Source: CAD feature listing. Evaluate the final solid. Frame: model axes, mm. A direction names the side the tool comes from. Coordinates: 2 decimals unless noted, no trailing zeros. Write each loop counter-clockwise with the first axis right and the second up, starting at its lowest first coordinate (ties: lowest second). Pieces come first, ordered by that corner, then holes. Notation, with made-up numbers: (5.25, -20) -> (29.25, -20) arc R12 cw to (29.25, -4) -> close; hole circle Ø10 at (-22.75, 49). An arc over 180 degrees is marked (long way). Write item = value, one per line.
from build123d import *

# Parameters (mm, degrees)
CUT_EXTRUDE_START   = -0.5
CUT_EXTRUDE_1_DEPTH = 6.83442973
CHAMFER_1_SIZE      = 0.2


with BuildPart() as part:
    # 草图1 → 旋转1 (revolve)
    with BuildSketch(Plane.XY, mode=Mode.PRIVATE) as revolve_1_sk:
        with BuildLine():
            Line((1.2, 2.75), (1.9, 2.75))
            Line((1.9, 2.75), (1.9, 1.5))
            Line((1.9, 1.5), (6.9, 1.5))
            Line((6.9, 1.5), (6.9, 0))
            Line((6.9, 0), (0, 0))
            ThreePointArc((0, 0), (0.313064269, 1.500208319), (1.2, 2.75))
        make_face()
    revolve(revolve_1_sk.sketch.rotate(Axis((0, 0, 0), (1, 0, 0)), 90), axis=Axis((0, 0, 0), (1, 0, 0)))

    # 草图2 → 切除-拉伸1 (cut, through all)
    with BuildSketch(Plane(origin=(1.9, 0, 0), x_dir=(0, 0, -1), z_dir=(1, 0, 0)).offset(CUT_EXTRUDE_START)):
        Polygon((0.35, -0.35), (0.35, -1.5), (-0.35, -1.5), (-0.35, -0.35), (-1.5, -0.35), (-1.5, 0.35), (-0.35, 0.35), (-0.35, 1.5), (0.35, 1.5), (0.35, 0.35), (1.5, 0.35), (1.5, -0.35), align=None)
    extrude(amount=-CUT_EXTRUDE_1_DEPTH, mode=Mode.SUBTRACT)

    # 草图3 → 旋转3 (revolve)
    with BuildSketch(Plane.XY, mode=Mode.PRIVATE) as revolve_3_sk:
        Polygon((1.9, 0), (1.9, 2), (0.9, 2), (1.4, 0), align=None)
    revolve(revolve_3_sk.sketch.rotate(Axis((0, 0, 0), (1, 0, 0)), 13.134022306), axis=Axis((0, 0, 0), (1, 0, 0)))

    # 倒角1
    chamfer_1_edges = [part.edges().sort_by_distance(p)[0] for p in [
        (6.9, 0, -1.5),
    ]]
    chamfer(chamfer_1_edges, length=CHAMFER_1_SIZE)


solid = part.part
1) Cut plane B-B, the plane z = -1.95. Output: boundary loops of the cut face in (x, y).
Answer block:
outline = (1.2, -1.94) -> (1.9, -1.94) -> (1.9, 1.94) -> (1.2, 1.94) arc R3.2 ccw to start
2) Reachability of faces 4 (the cylindrical face through (4.33, -0.45, 1.43)), 5 (the flat face through (0.7, 0.9, -0.35)) from +Z, -Z, +X, -X, +Y, -Y: full face, straight path, thin tool, end or side. Return the list, or none.
Answer block:
face_4 = +X
face_5 = -X
3) Material intervals for probe 1 along Z at (x, y) = (3.25, 0.8); probe 2 along Z at (x, y) = (6.25, -1.05); probe 3 along X at (y, z) = (-0.3, 0.1), sorted ascending. Write a range as [from, to].
Answer block:
probe_1 = [-1.27, 1.27]
probe_2 = [-1.07, 1.07]
probe_3 = [1.32, 6.9]
4) Cut plane A-A, the plane x = 4. Output: boundary loops of the cut face in (y, z).
Answer block:
outline = circle Ø3 at (0, 0)
5) Pull-direction query (Y, two-part tool) for faces 1 (the flat face through (0.7, 0.35, 0.9)), 2 (the cylindrical face through (1.555, 2.685, -0.596)), 3 (the flat face through (6.9, 0, 0)); classes: +Y half, -Y half, draft (parallel to the pull), parting line (faces both ways), or undercut.
Answer block:
face_1 = undercut
face_2 = parting line
face_3 = draft
6) First-contact query: pin 1 Ø1.3 at (x, z) = (0.5, 1) entering from +Y; pin 2 Ø1.3 at (x, z) = (1, -1) entering from +Y; pin 3 Ø0.8 at (x, y) = (0.5, 0) entering from +Z. Flat tips, straight axial feed; report the tip coordinate or a pass-through.
Answer block:
pin_1 = 2.55
pin_2 = 2.72
pin_3 = 2.44
7) Cut plane C-C, the plane y = -2.05. Output: boundary loops of the cut face in (x, z).
Answer block:
outline = (1.2, -1.83) -> (1.9, -1.83) -> (1.9, 1.83) -> (1.2, 1.83) arc R3.14 ccw to start
